Can you work these out from the drawing? Everything is in mm from the part's minimum corner. Give positions to 0.01 mm unless a question says otherwise; leave off trailing zeros. Order: outer loops, then holes, each group sorted by start corner. A loop starts at its lowest first (then second) coordinate and runs counter-clockwise, first axis right, second up. Notation, with made-up numbers: M -28,69 L 12,69 A24 ccw 12,96 Z; hole C 36.25,-11.75 d5. An arc over 180 degrees is marked long. Use a Markdown table: item, result. Add a question column.
Item 1: Suppose I cut it at C-C on x = 39.9. Write out the boundary of the cut face in (y, z).
Item 2: If I drill on L1, parallel to X at y = 34, z = 0.9; L2, parallel to Y at x = 19.5, z = 0.6; L3, parallel to Y at x = 52, z = 0.9, over which ranges is the centre line in solid material (lowest first)? Write a range as from..to.
Item 3: Suppose I cut it at A-A on y = 19.25. Write out the boundary of the cut face in (x, z), plus the area to 3 significant figures.
Item 4: I'm going to push a flat-ended pin straight in: pin 1 Ø4.5 at (x, y) = (50.1, 19.25) entering from +Z. Where does the tip first touch, or does it pass through?
Item 5: Suppose I cut it at D-D on x = 69. Write out the boundary of the cut face in (y, z), plus the area to 3 significant figures.
Item 6: Suppose I cut it at B-B on z = 0.85. Count the separate pieces of the cut face and the enclosed holes in it, plus the area to 3 significant figures.
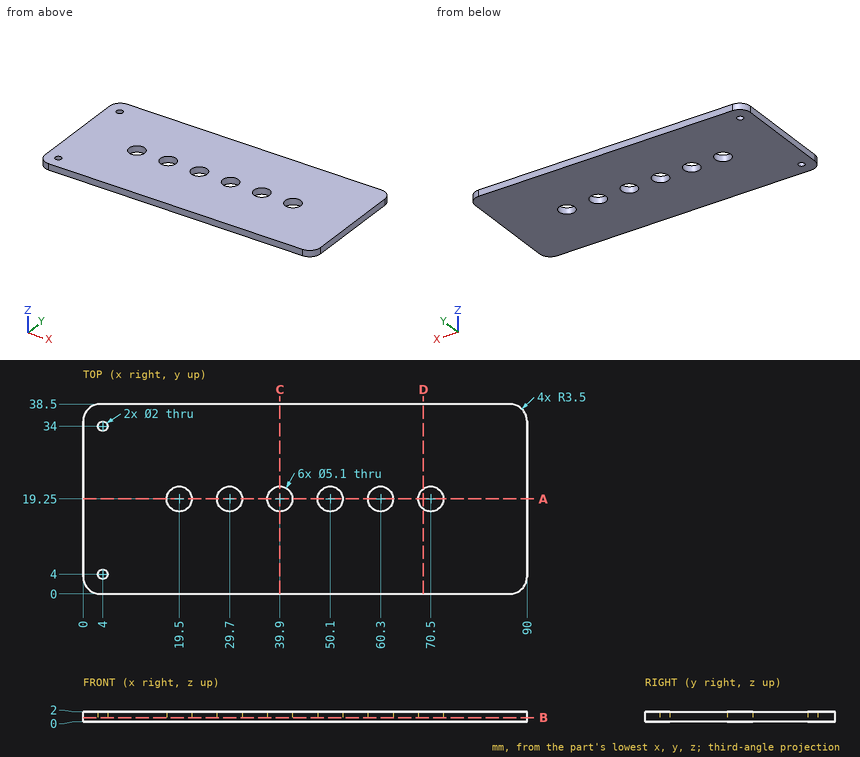
Findings below:
| question | item | result |
|---|---|---|
| 1 | outline | M 0,0 L 16.7,0 L 16.7,2 L 0,2 Z; M 21.8,0 L 38.5,0 L 38.5,2 L 21.8,2 Z |
| 2 | L1 | x = 0..3, 5..90 |
| 2 | L2 | y = 0..16.7, 21.8..38.5 |
| 2 | L3 | y = 0..17.55, 20.95..38.5 |
| 3 | outline | M 0,0 L 16.95,0 L 16.95,2 L 0,2 Z; M 22.05,0 L 27.15,0 L 27.15,2 L 22.05,2 Z; M 32.25,0 L 37.35,0 L 37.35,2 L 32.25,2 Z; M 42.45,0 L 47.55,0 L 47.55,2 L 42.45,2 Z; M 52.65,0 L 57.75,0 L 57.75,2 L 52.65,2 Z; M 62.85,0 L 67.95,0 L 67.95,2 L 62.85,2 Z; M 73.05,0 L 90,0 L 90,2 L 73.05,2 Z |
| 3 | area | 119 mm^2 |
| 4 | pin 1 | passes through |
| 5 | outline | M 0,0 L 17.19,0 L 17.19,2 L 0,2 Z; M 21.31,0 L 38.5,0 L 38.5,2 L 21.31,2 Z |
| 5 | area | 68.8 mm^2 |
| 6 | separate pieces | 1 |
| 6 | enclosed holes | 8 |
| 6 | area | 3,330 mm^2 |
